Design review of the part built by this model. Coordinates are the model's own, in mm. Coordinates: 2 decimals unless noted, no trailing zeros. Loops run counter-clockwise (first coordinate to the right, second up) from the corner with the lowest first, then second, coordinate; pieces in that order, holes last.
from build123d import *

# Parameters (mm, degrees)
SKETCH1_R           = 1.9
BOSS_EXTRUDE1_DEPTH = 6.95
SKETCH2_OUTSIDE_W   = 7.558
SKETCH2_OUTSIDE_H   = 7.558
SKETCH2_OUTSIDE_R   = 1.5
CUT_EXTRUDE1_DEPTH  = 2.6
SKETCH3_R           = 1
CUT_EXTRUDE2_DEPTH  = 7.95


with BuildPart() as part:
    # Sketch1 → Boss-Extrude1 (new body)
    with BuildSketch(Plane(origin=(0, 0, 0), x_dir=(1, 0, 0), z_dir=(0, 1, 0))):
        Circle(SKETCH1_R)
    extrude(amount=BOSS_EXTRUDE1_DEPTH)

    # Sketch2 outside → Cut-Extrude1 (cut)
    with BuildSketch(Plane(origin=(0, 6.95, 0), x_dir=(1, 0, 0), z_dir=(0, 1, 0))):
        Rectangle(SKETCH2_OUTSIDE_W, SKETCH2_OUTSIDE_H)
        Circle(SKETCH2_OUTSIDE_R, mode=Mode.SUBTRACT)
    extrude(amount=-CUT_EXTRUDE1_DEPTH, mode=Mode.SUBTRACT)

    # Sketch3 → Cut-Extrude2 (cut, through all)
    with BuildSketch(Plane.XZ):
        Circle(SKETCH3_R)
    extrude(amount=-CUT_EXTRUDE2_DEPTH, mode=Mode.SUBTRACT)


solid = part.part
Q1. For line 1 (Z direction, x = 0, y = 3.75); line 2 (Z direction, x = 0, y = 5.5); line 3 (X direction, y = 2.5, z = 0.15), list the stretches that pass through material, from the lowest coordinate up.
Q2. Take a section at A-A, the plane x = 0. Write out the cut boundary in (y, z).
Q3. The part is to be moulded in two halves that separate along Z. For faces 1 (the cylindrical face through (-1.5, 5.67, -0.07)), 2 (the cylindrical face through (0, 3, -1)), 3 (the flat face through (1, 0, 1)), say which applies: pulls with the +Z half, pulls with the -Z half, needs draft (parallel to the pull), parting line crosses it, or undercut.
Q4. Take a section at C-C, the plane y = 6. Write out the cut boundary in (x, z), then the cut area to 3 significant figures.
Q5. Take a section at B-B, the plane z = 0. Write out the cut boundary in (x, y).
Q6. Clearance check with a flat-ended pin moving along its axis: pin 1 Ø1 at (x, z) = (1, 0) entering from -Y. State where the tip first meets the part, or that it passes through.
Q7. Take a section at D-D, the plane z = -1.2. Write out the cut boundary in (x, y).
Entries:
1. line 1: z = -1.9 to -1, 1 to 1.9
1. line 2: z = -1.5 to -1, 1 to 1.5
1. line 3: x = -1.89 to -0.99, 0.99 to 1.89
2. outline: (0, -1.9) - (4.35, -1.9) - (4.35, -1.5) - (6.95, -1.5) - (6.95, -1) - (0, -1) - close; (0, 1) - (6.95, 1) - (6.95, 1.5) - (4.35, 1.5) - (4.35, 1.9) - (0, 1.9) - close
3. face 1: parting line crosses it
3. face 2: undercut
3. face 3: needs draft
4. outline: circle Ø3 at (0, 0); hole circle Ø2 at (0, 0)
4. area: 3.93 mm2
5. outline: (-1.9, 0) - (-1, 0) - (-1, 6.95) - (-1.5, 6.95) - (-1.5, 4.35) - (-1.9, 4.35) - close; (1, 0) - (1.9, 0) - (1.9, 4.35) - (1.5, 4.35) - (1.5, 6.95) - (1, 6.95) - close
6. pin 1: stops at y = 0
7. outline: (-1.47, 0) - (1.47, 0) - (1.47, 4.35) - (0.9, 4.35) - (0.9, 6.95) - (-0.9, 6.95) - (-0.9, 4.35) - (-1.47, 4.35) - close
